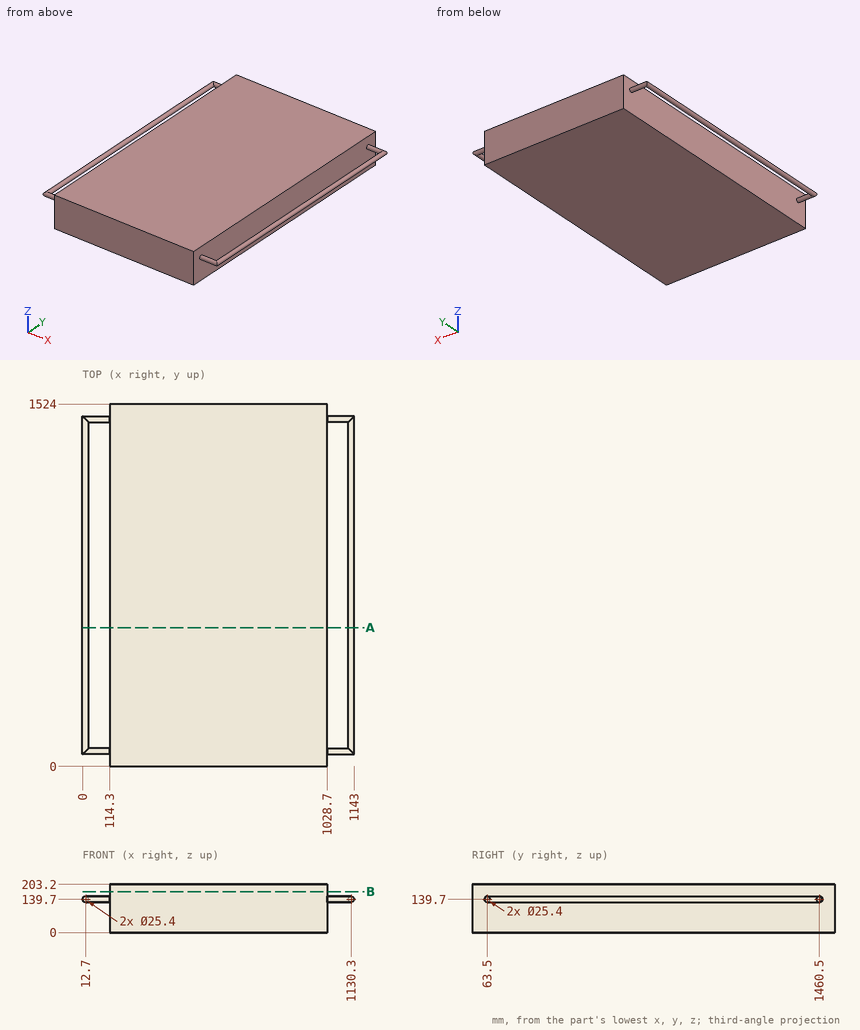
Study the drawing (mm; zero at the part's minimum x, y, z) and answer. Give positions to 0.01 mm unless a question says otherwise; leave off trailing zeros. Order: outer loops, then holes, each group sorted by start corner. A loop starts at its lowest first (then second) coordinate and runs counter-clockwise, first axis right, second up. Notation, with made-up numbers: (12.25, 49.5) - (25.25, 49.5) arc R22 ccw to (25.25, 58.5) - close; hole circle Ø5 at (-28, 47.5). An arc over 180 degrees is marked (long way). Answer in a Markdown table with one row per item. Add a question column.
Q1. Find the intervals of material crossed by line 1 along X through (y, z) = (864, 144.5); line 2 along X through (y, z) = (271, 19); line 3 along X through (y, z) = (178.5, 146), in increasing order. Write a range as [from, to].
Q2. Given P1, Ø4, axis at y = 1072, z = 131, coming from the +X side; P2, Ø8, axis at y = 1368, z = 61.5, coming from the +X side; P3, Ø1, axis at y = 157.5, z = 66, coming from the -X side, each flat-ended and moving along its own axis, determine where each tip first touches the part or whether it passes through.
Q3. The part is cut by section B-B (z = 172). Determine the outline of the cut face in (x, y).
Q4. The part is cut by section A-A (y = 583). Determine the outline of the cut face in (x, z).
Determined:
| question | item | result |
|---|---|---|
| 1 | line 1 | x = [0.94, 24.46], [114.3, 1028.7], [1118.54, 1142.06] |
| 1 | line 2 | x = [114.3, 1028.7] |
| 1 | line 3 | x = [1.67, 23.73], [114.3, 1028.7], [1119.27, 1141.33] |
| 2 | P1 | stops at x = 1141.09 |
| 2 | P2 | stops at x = 1028.7 |
| 2 | P3 | stops at x = 114.3 |
| 3 | outline | (114.3, 0) - (1028.7, 0) - (1028.7, 1524) - (114.3, 1524) - close |
| 4 | outline | circle Ø25.4 at (12.7, 139.7); (114.3, 0) - (1028.7, 0) - (1028.7, 203.2) - (114.3, 203.2) - close; circle Ø25.4 at (1130.3, 139.7) |
